The model under review builds one solid part; all positions refer to its coordinate system, in mm. Round coordinates to 2 decimals unless told otherwise and drop trailing zeros. Order: outer loops, then holes, each group sorted by start corner. A loop starts at its lowest first (then second) coordinate and runs counter-clockwise, first axis right, second up.
```python
from build123d import *

# Parameters (mm, degrees)
SKETCH1_W           = 50.84
SKETCH1_H           = 38.1
SKETCH1_R           = 1
SKETCH1_R_2         = 1.5
BOSS_EXTRUDE1_DEPTH = 1.6


with BuildPart() as part:
    # Sketch1 → Boss-Extrude1 (new body)
    with BuildSketch(Plane.XY):
        Rectangle(SKETCH1_W, SKETCH1_H)
        with Locations((-21.083254593, 15.8)):
            Circle(SKETCH1_R, mode=Mode.SUBTRACT)
        with Locations(Location((21.083254593, 15.8, 0), (0, 0, 180))):
            Circle(SKETCH1_R, mode=Mode.SUBTRACT)
        with Locations((21.083254593, -15.8)):
            Circle(SKETCH1_R, mode=Mode.SUBTRACT)
        with Locations(Location((-21.083254593, -15.8, 0), (0, 0, 180))):
            Circle(SKETCH1_R, mode=Mode.SUBTRACT)
        with Locations((-20.32, 0)):
            Circle(SKETCH1_R_2, mode=Mode.SUBTRACT)
        with Locations(Location((20.32, 0, 0), (0, 0, 180))):
            Circle(SKETCH1_R_2, mode=Mode.SUBTRACT)
    extrude(amount=BOSS_EXTRUDE1_DEPTH)


solid = part.part
```
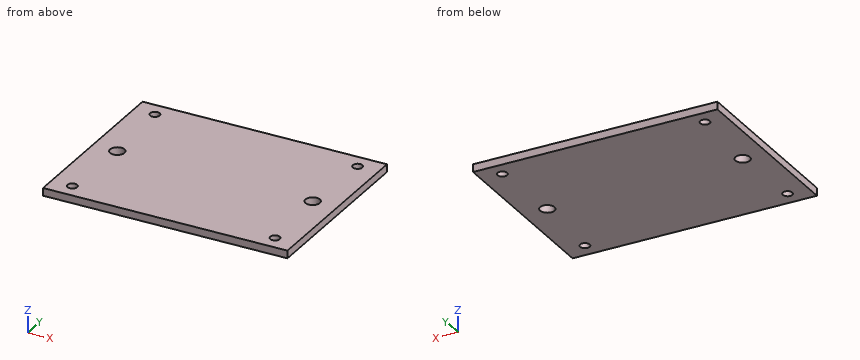
(1) Consider section A-A (y = 15.8). Write out the cut boundary in (x, z), and give its area (3 significant figures).
Data:
outline: (-25.42, 0) - (-22.08, 0) - (-22.08, 1.6) - (-25.42, 1.6) - close; (-20.08, 0) - (20.08, 0) - (20.08, 1.6) - (-20.08, 1.6) - close; (22.08, 0) - (25.42, 0) - (25.42, 1.6) - (22.08, 1.6) - close
area: 74.9 mm2
(2) Insertion check: pin 1 (3 mm diameter, centred on x = -21.08, y = -15.8, fed in from -Z). The pin has a flat end and moves straight along its axis. Give the tip position at first contact, or say it passes through.
Data:
pin 1: stops at z = 0
(3) To check wall thickness, follow probe 1 along Y at (x, z) = (21.5, 1.2); probe 2 along X at (y, z) = (0.5, 1.5); probe 3 along Y at (x, z) = (-20.32, 1.1). State the ranges of each line that lie inside material, in increasing order.
Data:
probe 1: y = -19.05 to -16.71, -14.89 to -0.93, 0.93 to 14.89, 16.71 to 19.05
probe 2: x = -25.42 to -21.73, -18.91 to 18.91, 21.73 to 25.42
probe 3: y = -19.05 to -16.45, -15.15 to -1.5, 1.5 to 15.15, 16.45 to 19.05
